Check sheet for the drawn part. Datum: minimum x, y, z corner. Units: mm. A direction names the side the tool comes from. Round coordinates to 2 decimals unless told otherwise and drop trailing zeros. Write each loop counter-clockwise with the first axis right and the second up, starting at its lowest first coordinate (ties: lowest second). Pieces come first, ordered by that corner, then holes.
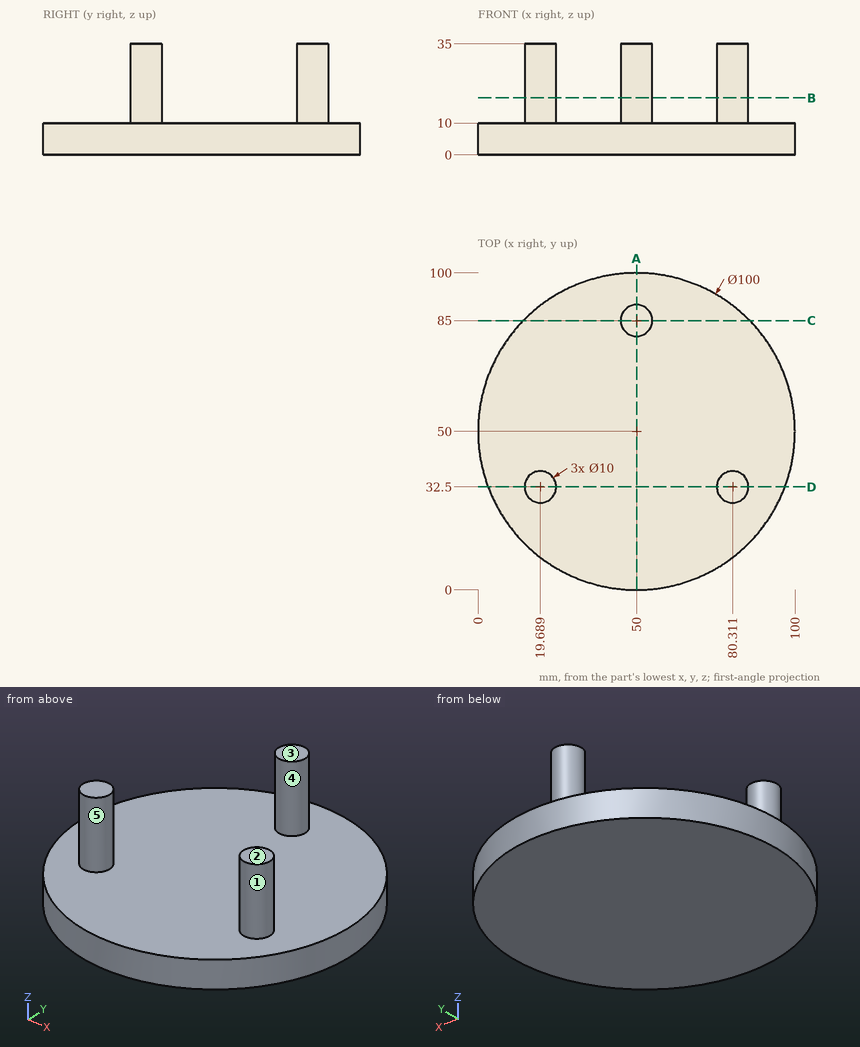
Q1. Sectioned sample at D-D (y = 32.5). Enter the section's corners in (x, z).
Recorded:
outline: (3.16, 0) - (96.84, 0) - (96.84, 10) - (85.31, 10) - (85.31, 35) - (75.31, 35) - (75.31, 10) - (24.69, 10) - (24.69, 35) - (14.69, 35) - (14.69, 10) - (3.16, 10) - close
Q2. Release check for a two-part mould opening along X. For the marked faces 3, 4 and 5 record: released by +X, released by -X, zero draft, split by the parting line, or undercut.
Recorded:
face 3: zero draft
face 4: split by the parting line
face 5: undercut
Q3. Material ranges on line 1 along Z through (x, y) = (7, 68); line 2 along Y through (x, z) = (36, 2.5); line 3 along X through (y, z) = (41.5, 7), recorded low to high.
Recorded:
line 1: z = 0 to 10
line 2: y = 2 to 98
line 3: x = 0.73 to 99.27
Q4. Sectioned sample at C-C (y = 85). Enter the section's corners in (x, z), plus the area to 3 significant figures.
Recorded:
outline: (14.29, 0) - (85.71, 0) - (85.71, 10) - (55, 10) - (55, 35) - (45, 35) - (45, 10) - (14.29, 10) - close
area: 964 mm2
Q5. Depth check by flat-ended pin: P1, Ø12, axis at x = 69, y = 24, coming from the +Z side; P2, Ø4, axis at y = 63.5, z = 10, coming from the -X side; P3, Ø8, axis at x = 79.5, z = 11, coming from the +Y side. Enter the tip coordinate at first touch or a pass-through.
Recorded:
P1: stops at z = 10
P2: stops at x = 1.34
P3: stops at y = 92.93
Q6. Sectioned sample at A-A (x = 50). Enter the section's corners in (y, z).
Recorded:
outline: (0, 0) - (100, 0) - (100, 10) - (90, 10) - (90, 35) - (80, 35) - (80, 10) - (0, 10) - close
Q7. Sectioned sample at B-B (z = 18). Enter the section's corners in (x, y), plus the area to 3 significant figures.
Recorded:
outline: circle Ø10 at (19.69, 32.5); circle Ø10 at (50, 85); circle Ø10 at (80.31, 32.5)
area: 236 mm2
Q8. Tool access check on the marked faces 1 and 2. Record the directions out of +Z, -Z, +X, -X, +Y, -Y that give a thin tool (end or side, any length) a straight path to the whole face; none if there is none.
Recorded:
face 1: +Z
face 2: +Z, +X, -X, +Y, -Y
